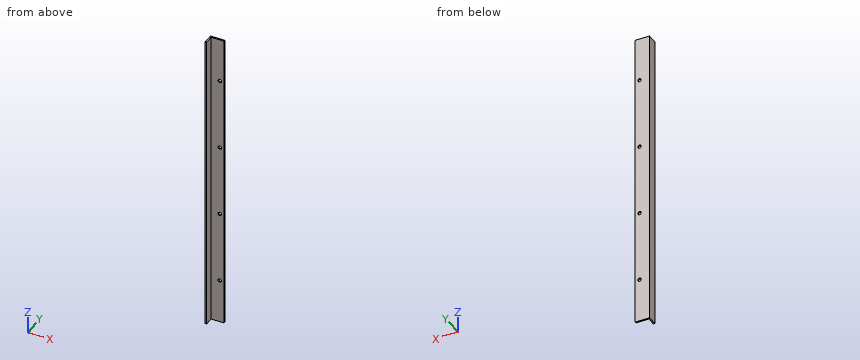
from build123d import *

# Parameters (mm, degrees)
EXTRUDE_1_DEPTH       = 212
HOLE_WIZARD_M21_D     = 2.4
HOLE_WIZARD_M21_DEPTH = 5
HOLE_WIZARD_M21_TIP   = 0.721032743


with BuildPart() as part:
    # Эскиз1 → Бобышка-Вытянуть1 (new body)
    with BuildSketch(Plane.XY):
        Polygon((0, 0), (0, 7), (10, 7), (10, 6), (1, 6), (1, 0), align=None)
    extrude(amount=EXTRUDE_1_DEPTH)

    # Отверстие с зазором M21
    with Locations(Plane(origin=(0, 7, 0), x_dir=(-1, 0, 0), z_dir=(0, 1, 0))):
        with Locations((-7, 131), (-7, 81), (-7, 31), (-7, 181)):
            Hole(HOLE_WIZARD_M21_D / 2, depth=HOLE_WIZARD_M21_DEPTH)
            with Locations((0, 0, -(HOLE_WIZARD_M21_DEPTH + HOLE_WIZARD_M21_TIP / 2))):  # 118° drill point
                Cone(0, HOLE_WIZARD_M21_D / 2, HOLE_WIZARD_M21_TIP, mode=Mode.SUBTRACT)


solid = part.part
Geometry: final body of the model. Coordinates: model frame, mm. Give positions to 0.01 mm unless a question says otherwise; leave off trailing zeros. Write each loop counter-clockwise with the first axis right and the second up, starting at its lowest first coordinate (ties: lowest second). Pieces come first, ordered by that corner, then holes.
(1) Ray query, line 1 (Z direction, x = 7, y = 6.55); line 2 (X direction, y = 6.45, z = 181); line 3 (X direction, y = 3, z = 72.5). Return the intervals inside material, ascending.
(2) Cut plane B-B, the plane y = 2.25. Return loops of the section in (x, z), then the cut area to 3 significant figures.
(3) Cut plane A-A, the plane z = 177. Return loops of the section in (x, y), then the cut area to 3 significant figures.
(4) First-contact query: P1, Ø3, axis at y = 2.5, z = 97, coming from the +X side; P2, Ø2, axis at x = 7, z = 181, coming from the +Y side; P3, Ø1, axis at x = 5.5, z = 43.5, coming from the -Y side; P4, Ø4, axis at y = 3.5, z = 97.5, coming from the -X side. Flat tips, straight axial feed; report the tip coordinate or a pass-through.
Values follow:
1. line 1: z = 0 to 29.8, 32.2 to 79.8, 82.2 to 129.8, 132.2 to 179.8, 182.2 to 212
1. line 2: x = 0 to 5.8, 8.2 to 10
1. line 3: x = 0 to 1
2. outline: (0, 0) - (1, 0) - (1, 212) - (0, 212) - close
2. area: 212 mm2
3. outline: (0, 0) - (1, 0) - (1, 6) - (10, 6) - (10, 7) - (0, 7) - close
3. area: 16.0 mm2
4. P1: stops at x = 1
4. P2: passes through
4. P3: stops at y = 6
4. P4: stops at x = 0
